Here's how the part is built. I have some questions about the finished solid (model axes, mm). Face numbers are marked on the shaded views. A direction names the side the tool comes from. Give positions to 0.01 mm unless a question says otherwise; leave off trailing zeros. Write each loop counter-clockwise with the first axis right and the second up, starting at its lowest first coordinate (ties: lowest second). Pieces come first, ordered by that corner, then holes. Notation, with made-up numbers: (-1.75, 88) -> (53.25, 88) arc R24 cw to (53.25, 116) -> close; hole circle Ø11 at (25.5, 11.25). An arc over 180 degrees is marked (long way). Use CSV: the item, a comma, the result in double quotes. Start each with the question number.
(1) If we mould it in two halves opening along X, with no side actions, what happens to the marked faces 1, 2, 3 and 4? For each: pulls with the +X half, pulls with the -X half, needs draft (parallel to the pull), parting line crosses it, or undercut.
(2) For pin 1 Ø5 at (x, z) = (16.5, 21) entering from -Y; pin 2 Ø0.9 at (x, y) = (18, 16) entering from -Z; pin 3 Ø7 at (y, z) = (19, 17.5) entering from -X; pin 4 Ø1.9 at (y, z) = (16.5, 6.5) entering from -X, each with a flat end and sliding along its axis, tell me the tip position at first contact or that it passes through.
(3) I need wall thicknesses on L1, parallel to Z at x = 6.5, y = 0.7; L2, parallel to Z at x = 15.5, y = 15.75; L3, parallel to X at y = 24, z = 8.5. Which ranges of each line are inside material? Lowest first, please. Write a range as [from, to].
(4) Suppose I cut it at A-A on x = 6.5. List the corners of the cut face in (y, z) for me, plus the area to 3 significant figures.
(5) Suppose I cut it at D-D on y = 18. List the corners of the cut face in (x, z) for me.
(6) Which directions (+Z, -Z, +X, -X, +Y, -Y) give clear straight access to the entire face, cutting with the end or side of a thin tool? Please do the marked faces 5 and 6.
(7) Suppose I cut it at C-C on z = 18.8. List the corners of the cut face in (x, y) for me, plus the area to 3 significant figures.
(8) Suppose I cut it at B-B on y = 2.5. List the corners of the cut face in (x, z) for me.
from build123d import *

# Parameters (mm, degrees)
BOSS_EXTRUDE1_DEPTH                       = 26
BLTOUCHPROBEMOUNTHOLESSKETCH2_R           = 2.05
BLTOUCHPROBEMOUNTHOLESCUT_EXTRUDE1_DEPTH  = 41.829033787
FILLET1_R                                 = 3
PROBESLIDINGMOUNTCUT_EXTRUDE3_DEPTH       = 42.117028103
PROBESLIDINGMOUNTCHANELCUT_EXTRUDE4_DEPTH = 1
CABLECHANNELSKETCH1_W                     = 5.5
CABLECHANNELSKETCH1_H                     = 28.1
CABLECUT_EXTRUDE1_DEPTH                   = 1.5


with BuildPart() as part:
    # ProfileSketch1 → Boss-Extrude1 (new body)
    with BuildSketch(Plane.XY):
        Polygon((0, 0), (19, 0), (19, 28.1), (15, 28.1), (15, 3), (0, 3), align=None)
    extrude(amount=BOSS_EXTRUDE1_DEPTH)

    # BLTouchProbeMountHolesSketch2 → BLTouchProbeMountHolesCut-Extrude1 (cut, through all)
    with BuildSketch(Plane(origin=(0, 3, 0), x_dir=(1, 0, 0), z_dir=(0, 1, 0))):
        with Locations(Location((6.5, -4, 0), (0, 0, 180))):
            Circle(BLTOUCHPROBEMOUNTHOLESSKETCH2_R)
        with Locations(Location((6.5, -22, 0), (0, 0, 180))):
            Circle(BLTOUCHPROBEMOUNTHOLESSKETCH2_R)
    extrude(amount=-BLTOUCHPROBEMOUNTHOLESCUT_EXTRUDE1_DEPTH, mode=Mode.SUBTRACT)

    # Fillet1
    fillet1_edges = [part.edges().sort_by_distance(p)[0] for p in [
        (19, 14.05, 26),
        (0, 1.5, 26),
        (19, 14.05, 0),
        (0, 1.5, 0),
    ]]
    fillet(fillet1_edges, radius=FILLET1_R)

    # ProbeSlidingMountSketch4 → ProbeSlidingMountCut-Extrude3 (cut, through all)
    with BuildSketch(Plane.ZY.offset(-15)):
        with BuildLine():
            Line((5.65, 19.9), (5.65, 10.9))
            ThreePointArc((5.65, 10.9), (7.2, 9.35), (8.75, 10.9))
            Line((8.75, 10.9), (8.75, 19.9))
            ThreePointArc((8.75, 19.9), (7.2, 21.45), (5.65, 19.9))
        make_face()
        with BuildLine():
            Line((17.25, 19.9), (17.25, 10.9))
            ThreePointArc((17.25, 10.9), (18.8, 9.35), (20.35, 10.9))
            Line((20.35, 10.9), (20.35, 19.9))
            ThreePointArc((20.35, 19.9), (18.8, 21.45), (17.25, 19.9))
        make_face()
    extrude(amount=-PROBESLIDINGMOUNTCUT_EXTRUDE3_DEPTH, mode=Mode.SUBTRACT)

    # ProbeSlidingMountChannelSketch5 → ProbeSlidingMountChanelCut-Extrude4 (cut)
    with BuildSketch(Plane.ZY.offset(-15)):
        with BuildLine():
            Line((10.4, 19.9), (10.4, 10.9))
            ThreePointArc((10.4, 10.9), (7.2, 7.7), (4, 10.9))
            Line((4, 10.9), (4, 19.9))
            ThreePointArc((4, 19.9), (7.2, 23.1), (10.4, 19.9))
        make_face()
        with BuildLine():
            Line((22, 19.9), (22, 10.9))
            ThreePointArc((22, 10.9), (18.8, 7.7), (15.6, 10.9))
            Line((15.6, 10.9), (15.6, 19.9))
            ThreePointArc((15.6, 19.9), (18.8, 23.1), (22, 19.9))
        make_face()
    extrude(amount=-PROBESLIDINGMOUNTCHANELCUT_EXTRUDE4_DEPTH, mode=Mode.SUBTRACT)

    # CableChannelSketch1 → CableCut-Extrude1 (cut)
    with BuildSketch(Plane(origin=(19, 0, 0), x_dir=(0, 0, -1), z_dir=(1, 0, 0))):
        with Locations((-13, 14.05)):
            Rectangle(CABLECHANNELSKETCH1_W, CABLECHANNELSKETCH1_H)
    extrude(amount=-CABLECUT_EXTRUDE1_DEPTH, mode=Mode.SUBTRACT)


solid = part.part
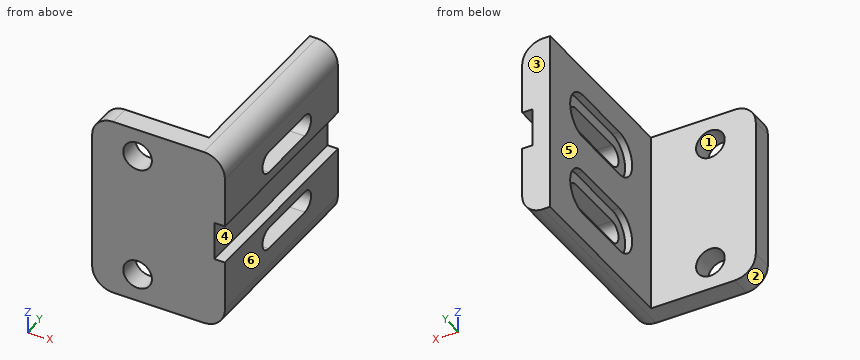
Geometry says:
1,face 1,"undercut"
1,face 2,"pulls with the -X half"
1,face 3,"needs draft"
1,face 4,"pulls with the +X half"
2,pin 1,"y = 0"
2,pin 2,"z = 0.43"
2,pin 3,"x = 15"
2,pin 4,"x = 16"
3,L1,"[0, 1.95], [6.05, 19.95], [24.05, 26]"
3,L2,"[0, 4], [10.4, 15.6], [22, 26]"
3,L3,"[15, 19]"
4,outline,"(0, 0) -> (3, 0) -> (3, 1.95) -> (0, 1.95) -> close; (0, 6.05) -> (3, 6.05) -> (3, 19.95) -> (0, 19.95) -> close; (0, 24.05) -> (3, 24.05) -> (3, 26) -> (0, 26) -> close"
4,area,"53.4 mm²"
5,outline,"(15, 0) -> (16, 0) arc R3 ccw to (19, 3) -> (19, 5.65) -> (16, 5.65) -> (16, 4) -> (15, 4) -> close; (15, 10.4) -> (16, 10.4) -> (16, 8.75) -> (19, 8.75) -> (19, 10.25) -> (17.5, 10.25) -> (17.5, 15.75) -> (19, 15.75) -> (19, 17.25) -> (16, 17.25) -> (16, 15.6) -> (15, 15.6) -> close; (15, 22) -> (16, 22) -> (16, 20.35) -> (19, 20.35) -> (19, 23) arc R3 ccw to (16, 26) -> (15, 26) -> close"
6,face 5,"+Z, -Z, -X, +Y"
6,face 6,"+Z, -Z, +X, +Y, -Y"
7,outline,"(0, 0) -> (19, 0) -> (19, 9.35) -> (16, 9.35) -> (16, 7.7) -> (15, 7.7) -> (15, 3) -> (0, 3) -> close; (15, 23.1) -> (16, 23.1) -> (16, 21.45) -> (19, 21.45) -> (19, 28.1) -> (15, 28.1) -> close"
7,area,"106 mm²"
8,outline,"(0, 3) arc R3 ccw to (3, 0) -> (16, 0) arc R3 ccw to (19, 3) -> (19, 10.25) -> (17.5, 10.25) -> (17.5, 15.75) -> (19, 15.75) -> (19, 23) arc R3 ccw to (16, 26) -> (3, 26) arc R3 ccw to (0, 23) -> close; hole circle Ø4.1 at (6.5, 4); hole circle Ø4.1 at (6.5, 22)"
